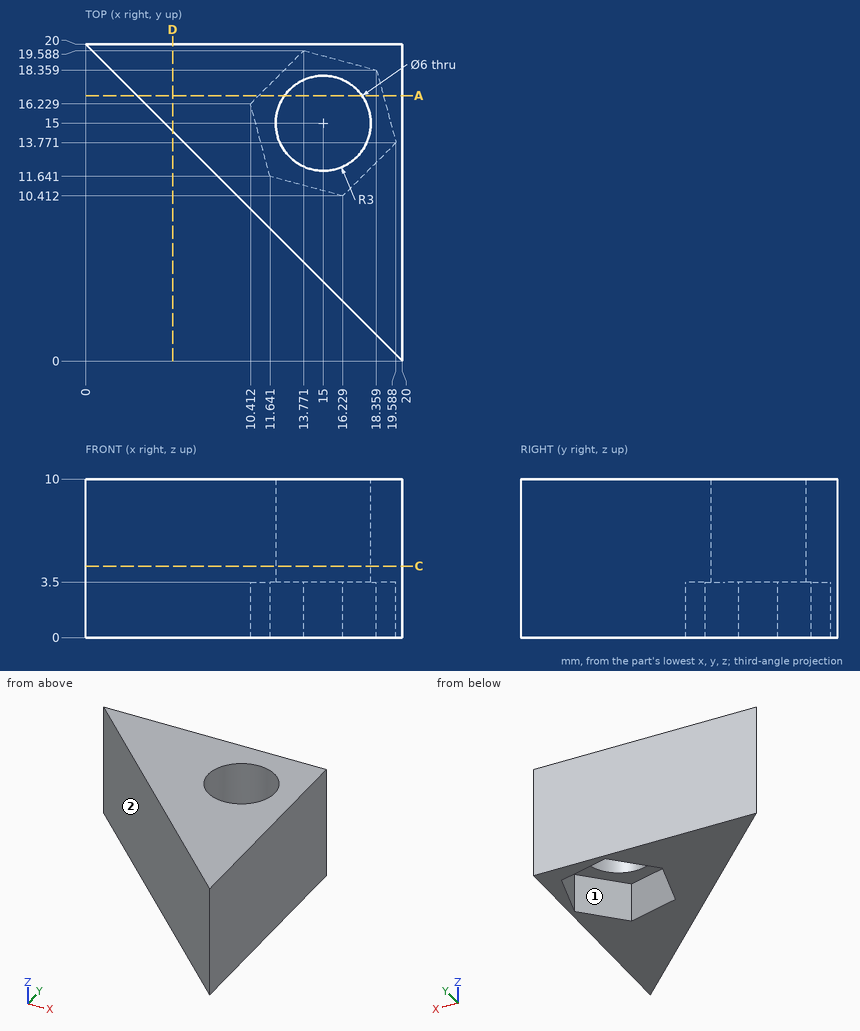
Can you work these out from the drawing? Everything is in mm from the part's minimum corner. A direction names the side the tool comes from. Round coordinates to 2 decimals unless told otherwise and drop trailing zeros. Loops run counter-clockwise (first coordinate to the right, second up) from the corner with the lowest first, then second, coordinate; pieces in that order, holes last. Notation, with made-up numbers: M 26.5,33.25 L 44.5,33.25 A16 ccw 44.5,64.25 Z; hole C 41.25,-5 d6. An arc over 180 degrees is marked long. Answer in a Markdown table with one row per item.
1. If we section it at A-A, the plane y = 16.75: Please give me the cut outline in (x, z).
Established:
| item | result |
|---|---|
| outline | M 3.25,0 L 10.93,0 L 10.93,3.5 L 12.56,3.5 L 12.56,10 L 3.25,10 Z; M 17.44,3.5 L 18.79,3.5 L 18.79,0 L 20,0 L 20,10 L 17.44,10 Z |
2. Please list where these lines run through material, in increasing order: line 1 (Y direction, x = 15, z = 7); line 2 (X direction, y = 17, z = 3.75) (1 decimal); line 3 (X direction, y = 13.5, z = 2.25) (1 decimal). Write a range as from..to.
Established:
| item | result |
|---|---|
| line 1 | 5..12, 18..20 |
| line 2 | 3..12.8, 17.2..20 |
| line 3 | 6.5..11.1, 19.3..20 |
3. I'm going to push a flat-ended pin straight in: pin 1 Ø2 at (x, y) = (15.5, 3) entering from -Z. Where does the tip first touch, or does it pass through?
Established:
| item | result |
|---|---|
| pin 1 | through |
4. If we section it at C-C, the plane z = 4.5: Please give me the cut outline in (x, y).
Established:
| item | result |
|---|---|
| outline | M 0,20 L 20,0 L 20,20 Z; hole M 12.88,12.88 A3 ccw 18,15 A3 ccw long Z |
5. On a 3-axis mill with a long thin cutter (end or side, diameter ignored), from which of +Z, -Z, +X, -X, +Y, -Y can I reach the whole of each face in a straight line? I mean the marked faces 1 and 2. Say none if no direction works.
Established:
| item | result |
|---|---|
| face 1 | -Z |
| face 2 | +Z, -Z, -X, -Y |
6. If we section it at D-D, the plane x = 5.5: Please give me the cut outline in (y, z).
Established:
| item | result |
|---|---|
| outline | M 14.5,0 L 20,0 L 20,10 L 14.5,10 Z |
